Here's how the part is built. I have some questions about the finished solid (model axes, mm). A direction names the side the tool comes from. Give positions to 0.01 mm unless a question says otherwise; leave off trailing zeros. Write each loop counter-clockwise with the first axis right and the second up, starting at its lowest first coordinate (ties: lowest second). Pieces come first, ordered by that corner, then holes. Notation, with made-up numbers: (-38.5, 51.5) - (16.5, 51.5) arc R27 cw to (16.5, 85.5) - close; hole circle Ø1 at (8, 85.25). An arc over 180 degrees is marked (long way). Use one line per item in the form item = value. Start each with the question number.
from build123d import *

# Parameters (mm, degrees)
BOSS_EXTRUDE1_DEPTH      = 50.8
F_5_16_CLEARANCE_HOLE3_D = 8.4328
CUT_EXTRUDE2_DEPTH       = 20.05
CUT_EXTRUDE2_DEPTH_BACK  = 20.05
F_5_16_CLEARANCE_HOLE2_D = 8.4328


with BuildPart() as part:
    # Sketch1 → Boss-Extrude1 (new body)
    with BuildSketch(Plane.XY):
        Polygon((-19.05, 0), (19.05, 0), (19.05, 50.8), (11.1125, 50.8), (11.1125, 6.35), (-11.1125, 6.35), (-11.1125, 50.8), (-19.05, 50.8), align=None)
    extrude(amount=BOSS_EXTRUDE1_DEPTH)

    # 5/16 Clearance Hole3 (through all)
    with Locations(Plane(origin=(0, 6.35, 0), x_dir=(1, 0, 0), z_dir=(0, 1, 0))):
        with Locations((0, -38.1), (0, -12.7)):
            Hole(F_5_16_CLEARANCE_HOLE3_D / 2)

    # Sketch18 → Cut-Extrude2 (cut, two sides)
    with BuildSketch(Plane(origin=(0, 0, 0), x_dir=(0, 0, -1), z_dir=(1, 0, 0))) as cut_extrude2_sk:
        with BuildLine():
            Line((0, 50.8), (-50.8, 50.8))
            Line((-50.8, 50.8), (-50.8, 28.575))
            ThreePointArc((-50.8, 28.575), (-41.91, 37.465), (-33.02, 28.575))
            ThreePointArc((-33.02, 28.575), (-28.370320151, 17.349679849), (-17.145, 12.7))
            Line((-17.145, 12.7), (-6.35, 12.7))
            ThreePointArc((-6.35, 12.7), (-1.859871939, 10.840128061), (0, 6.35))
            Line((0, 6.35), (0, 50.8))
        make_face()
    extrude(amount=CUT_EXTRUDE2_DEPTH, mode=Mode.SUBTRACT)
    extrude(cut_extrude2_sk.sketch, amount=-CUT_EXTRUDE2_DEPTH_BACK, mode=Mode.SUBTRACT)

    # 5/16 Clearance Hole2 (through all)
    with Locations(Plane(origin=(19.05, 0, 0), x_dir=(0, 0, -1), z_dir=(1, 0, 0))):
        with Locations((-41.91, 28.575)):
            Hole(F_5_16_CLEARANCE_HOLE2_D / 2)


solid = part.part
1. I want a section at D-D, the plane z = 7.5. List the corners of the cut face in (x, y) for me.
2. I want a section at A-A, the plane x = 0. List the corners of the cut face in (y, z) for me.
3. For faces 4 (the face through (-15, 12.7, 12)), 5 (the face through (0, 3, 0)), 6 (the face through (11.112, 15, 36)), which set-ups out of +Z, -Z, +X, -X, +Y, -Y let a thin tool reach every point of the face, with its end or its side?
4. I want a section at B-B, the plane y = 33.5. List the corners of the cut face in (x, z) for me, then the cut area to 3 significant figures.
5. Please list where these lines run through material, in increasing order: line 1 (Z direction, x = 0, y = 2.75); line 2 (X direction, y = 34.5, z = 47); line 3 (Y direction, x = -15.5, z = 41.91) (3 decimals).
6. For P1, Ø10, axis at x = -11.5, z = 34, coming from the +Y side; P2, Ø1.5, axis at x = -8.5, y = 25.5, coming from the +Z side; P3, Ø8.5, axis at x = -13.5, z = 9.5, coming from the +Y side; P4, Ø11, axis at x = -2, z = 31.5, coming from the +Y side, each with a flat end and sliding along its axis, tell me the tip position at first contact or that it passes through.
7. I want a section at C-C, the plane z = 14. List the corners of the cut face in (x, y) for me.
8. We'd pull the mould along Y, two halves only. Please class faces 1 (the face through (-15.137, 32.756, 41.361)), 2 (the face through (15.03, 17.47, 28.49)), 3 (the face through (0, 0, 25)): pulls with the +Y half, pulls with the -Y half, needs draft (parallel to the pull), parting line crosses it, or undercut.
Result sheet:
q1.outline = (-19.05, 0) - (19.05, 0) - (19.05, 12.7) - (11.11, 12.7) - (11.11, 6.35) - (-11.11, 6.35) - (-11.11, 12.7) - (-19.05, 12.7) - close
q2.outline = (0, 0) - (6.35, 0) - (6.35, 8.48) - (0, 8.48) - close; (0, 16.92) - (6.35, 16.92) - (6.35, 33.88) - (0, 33.88) - close; (0, 42.32) - (6.35, 42.32) - (6.35, 50.8) - (0, 50.8) - close
q3.face_4 = -Z, +X, -X, +Y
q3.face_5 = -Z, +X, -X, +Y, -Y
q3.face_6 = +Z, -Z, +Y
q4.outline = (-19.05, 34.51) - (-11.11, 34.51) - (-11.11, 49.31) - (-19.05, 49.31) - close; (11.11, 34.51) - (19.05, 34.51) - (19.05, 49.31) - (11.11, 49.31) - close
q4.area = 235 mm2
q5.line_1 = 0 to 8.48, 16.92 to 33.88, 42.32 to 50.8
q5.line_2 = -19.05 to -11.11, 11.11 to 19.05
q5.line_3 = 0 to 24.359, 32.791 to 37.465
q6.P1 = 36.98
q6.P2 = through
q6.P3 = 12.7
q6.P4 = 6.35
q7.outline = (-19.05, 0) - (-4.01, 0) - (-4.01, 6.35) - (-11.11, 6.35) - (-11.11, 12.7) - (-19.05, 12.7) - close; (4.01, 0) - (19.05, 0) - (19.05, 12.7) - (11.11, 12.7) - (11.11, 6.35) - (4.01, 6.35) - close
q8.face_1 = undercut
q8.face_2 = pulls with the +Y half
q8.face_3 = pulls with the -Y half
